Autodesk Inventor part; units mm, degrees
ref_plane "YZ Plane" through (0, 0, 0) normal (1, 0, 0) x (0, 1, 0)
ref_plane "XZ Plane" through (0, 0, 0) normal (0, 1, 0) x (-1, 0, 0)
ref_plane "XY Plane" through (0, 0, 0) normal (0, 0, 1) x (1, 0, 0)
sketch "Sketch1" plane through (0, 0, 0) normal (0, 0, 1) x (1, 0, 0)
  line L0 (-37.1688, 9.374) -> (-37.1688, 9.374)
  line L1 (-34.6288, 6.834) -> (-21.9288, 6.834)
  line L2 (-21.9288, 6.834) -> (-21.9288, 8.104)
  line L3 (-21.9288, 8.104) -> (-34.6288, 8.104)
  line L4 (-35.8988, 9.374) -> (-35.8988, 9.374)
  line L5 (-35.8988, 9.374) -> (-37.1688, 9.374)
  arc A0 (-35.8988, 9.374) -> (-34.6288, 8.104) centre (-34.6288, 9.374) ccw
  arc A1 (-37.1688, 9.374) -> (-34.6288, 6.834) centre (-34.6288, 9.374) ccw
  dimension "d0" = 1.27
  dimension "d1" = 1.27
  dimension "d2" = 2.54
  dimension "d3" = 1.27
  dimension "d4" = 15.24
  dimension "d5" = 2.54
extrude "Extrusion1" add sketch "Sketch1" along normal blind 6.35
sketch "Sketch2" plane through (-34.6288, 8.104, 0) normal (0, 1, 0) x (1, 0, 0)
  line L0 (0, -6.35) -> (12.7, -6.35)
  line L1 (0, 0) -> (12.7, 0)
  circle A0 centre (2.54, -3.175) radius 3.175 construction
  dimension "d8" = 10.16
hole "Hole1" at (-32.0888, 8.104, 3.175) at (-32.0888, 8.104, 3.175) direction (0, -1, 0) diameter 2.6416 end through all
sketch "Sketch3" plane through (-34.6288, 8.104, 0) normal (0, 1, 0) x (1, 0, 0)
  circle A0 centre (2.54, -3.175) radius 1.3208
  point P0 (8.89, -3.175)
  dimension "d16" = 6.35
hole "Hole2" at (-25.7388, 8.104, 3.175) direction (0, -1, 0) diameter 1.27 end through all
properties part number "contact" material "Brass, Soft Yellow"
Read the model definition and answer for the solid it produces. Units are mm, in the model's axes. A direction names the side the tool comes from. Round coordinates to 2 decimals unless told otherwise and drop trailing zeros. Write each loop counter-clockwise with the first axis right and the second up, starting at its lowest first coordinate (ties: lowest second). Pieces come first, ordered by that corner, then holes.
Q1. Flat-ended cylindrical pins translate along their axes: P1, Ø1.6, axis at x = -32.09, z = 3.18, coming from the -Y side; P2, Ø1.5, axis at y = 7.5, z = 4.5, coming from the -X side; P3, Ø2, axis at x = -25.74, z = 3.18, coming from the +Y side. Find the tip coordinate at first contact, or state that the pin passes through.
Values:
P1: passes through
P2: stops at x = -36.91
P3: stops at y = 8.1
Q2. A tool of negligible diameter and unlimited length cuts with its end or side. For faces 1 (the face through (-29.7, 7.6, 6.35)), 2 (the face through (-28, 8.104, 3)), from which of +Z, -Z, +X, -X, +Y, -Y can it reach the whole face along a straight path? Write none if from no direction.
Values:
face 1: +Z, +X, -X, +Y, -Y
face 2: +Z, -Z, +X, +Y
Q3. The mould has two halves that part along X. Classify faces 3 (the face through (-30.8, 7.46, 2.89)), 4 (the face through (-28, 6.834, 3)), 5 (the face through (-21.929, 7, 3)): released by +X, released by -X, zero draft, split by the parting line, or undercut.
Values:
face 3: undercut
face 4: zero draft
face 5: released by +X
Q4. Find section A-A on x = -32.5. Determine the outline of the cut face in (y, z).
Values:
outline: (6.83, 0) - (8.1, 0) - (8.1, 1.92) - (6.83, 1.92) - close; (6.83, 4.43) - (8.1, 4.43) - (8.1, 6.35) - (6.83, 6.35) - close
Q5. Straight lines are drawn through the part: line 1 (X direction, y = 8.05, z = 3.25); line 2 (X direction, y = 7.8, z = 3.25); line 3 (Y direction, x = -23.5, z = 6.25). For each, find the intervals that lie inside material, in ascending order.
Values:
line 1: x = -36.8 to -33.41, -30.77 to -26.37, -25.11 to -21.93
line 2: x = -36.62 to -33.41, -30.77 to -26.37, -25.11 to -21.93
line 3: y = 6.83 to 8.1
Q6. Find section C-C on y = 7.05. Determine the outline of the cut face in (x, z) (3 decimals), and give its area (3 significant figures).
Values:
outline: (-35.654, 0) - (-21.929, 0) - (-21.929, 6.35) - (-35.654, 6.35) - close; hole circle Ø2.642 at (-32.089, 3.175); hole circle Ø1.27 at (-25.739, 3.175)
area: 80.4 mm2
Q7. Find section B-B on z = 4.25. Determine the outline of the cut face in (x, y).
Values:
outline: (-37.17, 9.37) arc R2.54 ccw to (-34.63, 6.83) - (-32.86, 6.83) - (-32.86, 8.1) - (-34.63, 8.1) arc R1.27 cw to (-35.9, 9.37) - close; (-31.32, 6.83) - (-21.93, 6.83) - (-21.93, 8.1) - (-31.32, 8.1) - close
Q8. Find section D-D on z = 5.25. Determine the outline of the cut face in (x, y), and give its area (3 significant figures).
Values:
outline: (-37.17, 9.37) arc R2.54 ccw to (-34.63, 6.83) - (-21.93, 6.83) - (-21.93, 8.1) - (-34.63, 8.1) arc R1.27 cw to (-35.9, 9.37) - close
area: 19.9 mm2
